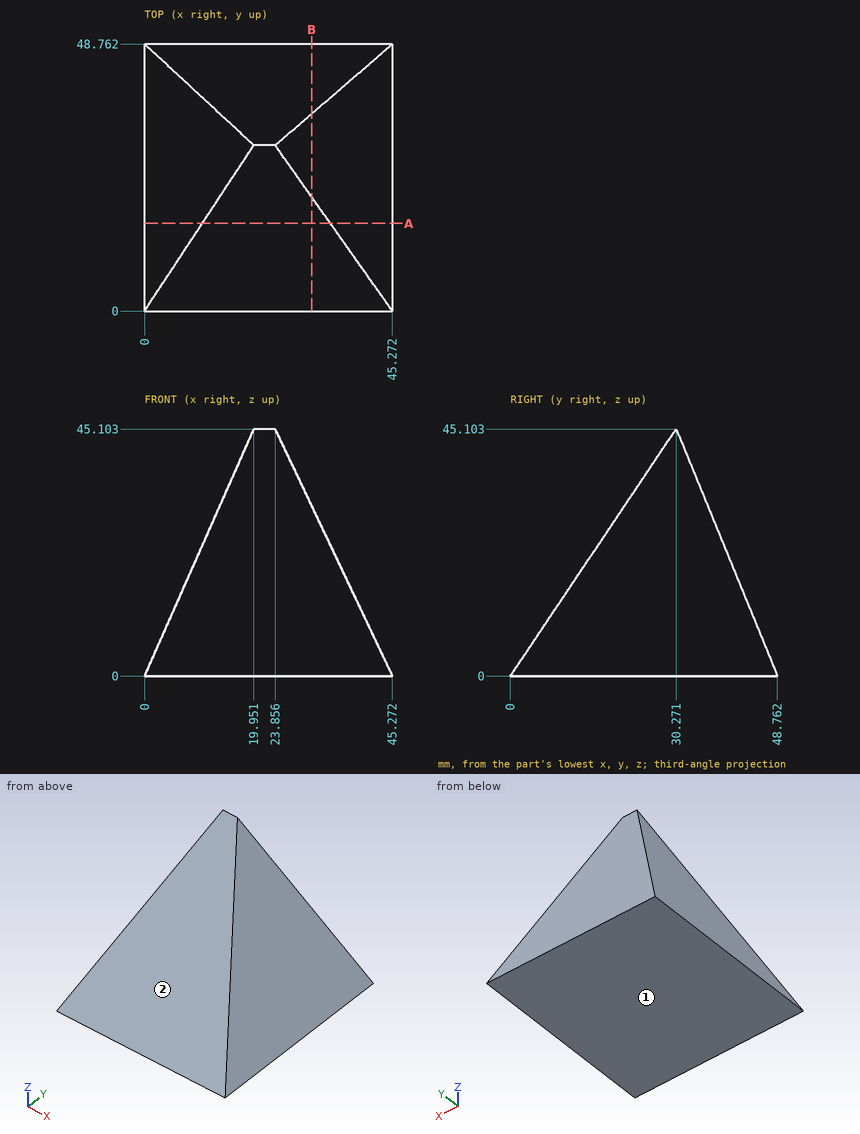
Design review of the part shown in the three views and the two pictorial views. Dimensions are in mm from the part's minimum x, y and z. Coordinates: 2 decimals unless noted, no trailing zeros. Loops run counter-clockwise (first coordinate to the right, second up) from the corner with the lowest first, then second, coordinate; pieces in that order, holes last.
Q1. To check wall thickness, follow line 1 (Z direction, x = 26.5, y = 22.5) (1 decimal); line 2 (Z direction, x = 8, y = 43.5) (1 decimal); line 3 (Y direction, x = 22, z = 23). State the ranges of each line that lie inside material, in increasing order.
Reported:
line 1: z = 0 to 33.5
line 2: z = 0 to 12.8
line 3: y = 15.44 to 39.33
Q2. For pin 1 (6 mm diameter, centred on y = 17.5, z = 36, fed in from -X); pin 2 (1 mm diameter, centred on x = 16, z = 23, fed in from +Y); pin 3 (4 mm diameter, centred on x = 18, y = 8.5, fed in from +Z) (1 decimal); pin 4 (1.5 mm diameter, centred on y = 24.5, z = 8, fed in from +X), all flat-tipped, find the tip position at first contact; note any pin that passes through.
Reported:
pin 1: passes through
pin 2: stops at y = 39.54
pin 3: stops at z = 15.6
pin 4: stops at x = 41.83
Q3. The part is to be moulded in two halves that separate along Z. For the marked faces 1 and 2, say which applies: +Z half, -Z half, draft (parallel to the pull), parting line (faces both ways), or undercut.
Reported:
face 1: -Z half
face 2: +Z half
Q4. We need section A-A on y = 16. State the section outline as (x, z) points (1 decimal).
Reported:
outline: (0, 0) - (45.3, 0) - (34, 23.8) - (10.5, 23.8) - close
Q5. We need section B-B on x = 30.5. State the section outline as (y, z) points, and give its area (3 significant figures).
Reported:
outline: (0, 0) - (48.76, 0) - (36.01, 31.11) - (20.88, 31.11) - close
area: 994 mm2
